For this review, take the finished solid that the model builds, in its own axes (mm). A direction names the side the tool comes from. Coordinates: 2 decimals unless noted, no trailing zeros. Loops run counter-clockwise (first coordinate to the right, second up) from the corner with the lowest first, then second, coordinate; pieces in that order, holes last. Notation, with made-up numbers: (80.5, 69) -> (104.5, 69) arc R24 cw to (104.5, 102) -> close; hole circle Ø8 at (2.25, 46.25). An arc over 180 degrees is marked (long way). Use a Markdown table: item, result.
from build123d import *

# Parameters (mm, degrees)
BLANKSKE_W          = 40
BLANKSKE_H          = 8.2
BLANK_DEPTH         = 5
TOOTHCUTILL_DEPTH   = 42.136844799
TOOTHCUTSIM_DEPTH   = 42.136844799
TEETHCUTS_COUNT     = 13
TEETHCUTS_PITCH     = 3.14159265
SKETCH1_W           = 4.99804548
SKETCH1_H           = 2.25
BOSS_EXTRUDE1_DEPTH = 5
SKETCH4_W           = 12
SKETCH4_H           = 2.25
BOSS_EXTRUDE4_DEPTH = 14.5
BOSS_EXTRUDE5_DEPTH = 2.75


with BuildPart() as part:
    # BlankSke → Blank (new body)
    with BuildSketch(Plane.XY):
        with Locations((20, 4.1)):
            Rectangle(BLANKSKE_W, BLANKSKE_H)
    extrude(amount=-BLANK_DEPTH)

    # TooCutSkeIll → ToothCutIll (cut, through all)
    with BuildSketch(Plane.XY):
        with BuildLine():
            Line((-1.253788993, 8.173680806), (-0.504546125, 6.115152944))
            ThreePointArc((-0.504546125, 6.115152944), (-0.412650963, 5.995392837), (-0.268683278, 5.95))
            Line((-0.268683278, 5.95), (0.268683278, 5.95))
            ThreePointArc((0.268683278, 5.95), (0.412650963, 5.995392837), (0.504546125, 6.115152944))
            Line((0.504546125, 6.115152944), (1.253788993, 8.173680806))
            ThreePointArc((1.253788993, 8.173680806), (1.268433641, 8.192766082), (1.291376698, 8.2))
            Line((1.291376698, 8.2), (1.291376698, 8.2254))
            Line((1.291376698, 8.2254), (-1.291376698, 8.2254))
            Line((-1.291376698, 8.2254), (-1.291376698, 8.2))
            ThreePointArc((-1.291376698, 8.2), (-1.268433641, 8.192766082), (-1.253788993, 8.173680806))
        make_face()
    toothcutill = extrude(amount=-TOOTHCUTILL_DEPTH, mode=Mode.SUBTRACT)

    # TooCutSkeSim → ToothCutSim (cut, through all)
    with BuildSketch(Plane.XY):
        Polygon((0.44443537, 5.95), (-0.44443537, 5.95), (-1.272613241, 8.2254), (1.272613241, 8.2254), align=None)
    toothcutsim = extrude(amount=-TOOTHCUTSIM_DEPTH, mode=Mode.SUBTRACT)

    # TeethCuts: ToothCutIll, ToothCutSim ×13
    with Locations(*[(i * TEETHCUTS_PITCH, 0, 0) for i in range(1, TEETHCUTS_COUNT)]):
        add(toothcutill, mode=Mode.SUBTRACT)
        add(toothcutsim, mode=Mode.SUBTRACT)

    # Sketch1 → Boss-Extrude1 (add)
    with BuildSketch(Plane.XY):
        with Locations((37.50097726, 7.075)):
            Rectangle(SKETCH1_W, SKETCH1_H)
    extrude(amount=-BOSS_EXTRUDE1_DEPTH)

    # Sketch4 → Boss-Extrude4 (add)
    with BuildSketch(Plane(origin=(40, 0, 0), x_dir=(0, 0, -1), z_dir=(1, 0, 0))):
        with Locations((6, 7.075)):
            Rectangle(SKETCH4_W, SKETCH4_H)
    extrude(amount=BOSS_EXTRUDE4_DEPTH)

    # Sketch6 → Boss-Extrude5 (add)
    with BuildSketch(Plane(origin=(0, 8.2, 0), x_dir=(1, 0, 0), z_dir=(0, 1, 0))):
        Polygon((35.00195452, 5), (35.00195452, 0), (54.5, 0), (54.5, 12), (40, 12), (40, 5), align=None)
    extrude(amount=BOSS_EXTRUDE5_DEPTH)


solid = part.part
(1) Mouldability with a two-part tool opening along X and no side actions: class faces 4 (the face through (47, 5.95, -6)), 5 (the face through (40, 3, -2)), 6 (the face through (12.6, 5.95, -2.5)) as pulls with the +X half, pulls with the -X half, needs draft (parallel to the pull), parting line crosses it, or undercut.
Found:
| item | result |
|---|---|
| face 4 | needs draft |
| face 5 | pulls with the +X half |
| face 6 | undercut |
(2) For faces 1 (the face through (0, 3, -2)), 2 (the face through (22, 5.95, -2)), 3 (the face through (20, 4, -5)), list the 3-axis set-ups (+Z, -Z, +X, -X, +Y, -Y) from which the entire face can be reached by the end or side of a thin tool; tool diameter is ignored.
Found:
| item | result |
|---|---|
| face 1 | +Z, -Z, -X, +Y, -Y |
| face 2 | +Z, -Z, +Y |
| face 3 | -Z, -X, +Y, -Y |
(3) Take a section at D-D on y = 6.75. State how many separate pieces and enclosed holes the cut face has, plus the area to 3 significant figures.
Found:
| item | result |
|---|---|
| separate pieces | 12 |
| enclosed holes | 0 |
| area | 291 mm^2 |
(4) Take a section at C-C on z = -10. Write out the cut boundary in (x, y).
Found:
| item | result |
|---|---|
| outline | (40, 5.95) -> (54.5, 5.95) -> (54.5, 10.95) -> (40, 10.95) -> close |
(5) For line 1 along Z through (x, y) = (7.5, 7); line 2 along Y through (x, z) = (46, -5); line 3 along X through (y, z) = (6.25, -6.5), list the stretches that pass through material, from the lowest coordinate up.
Found:
| item | result |
|---|---|
| line 1 | z = -5 to 0 |
| line 2 | y = 5.95 to 10.95 |
| line 3 | x = 40 to 54.5 |
(6) Take a section at B-B on x = 48.5. Write out the cut boundary in (y, z), plus the area to 3 significant figures.
Found:
| item | result |
|---|---|
| outline | (5.95, -12) -> (10.95, -12) -> (10.95, 0) -> (5.95, 0) -> close |
| area | 60.0 mm^2 |
(7) For pin 1 Ø0.6 at (x, z) = (20.5, -3) entering from +Y; pin 2 Ø1.5 at (y, z) = (9.5, -1.5) entering from -X; pin 3 Ø2.5 at (y, z) = (4, -3) entering from +X, all flat-tipped, find the tip position at first contact; note any pin that passes through.
Found:
| item | result |
|---|---|
| pin 1 | stops at y = 8.2 |
| pin 2 | stops at x = 35 |
| pin 3 | stops at x = 40 |
(8) Take a section at A-A on y = 8.75. Write out the cut boundary in (x, z).
Found:
| item | result |
|---|---|
| outline | (35, -5) -> (40, -5) -> (40, -12) -> (54.5, -12) -> (54.5, 0) -> (35, 0) -> close |
